Could you check a few things on this model? Use its own coordinates, in mm. Face numbers are marked on the shaded views. Round coordinates to 2 decimals unless told otherwise and drop trailing zeros. Write each loop counter-clockwise with the first axis right and the second up, starting at its lowest first coordinate (ties: lowest second). Pieces come first, ordered by that corner, then holes. Notation, with made-up numbers: (-37, 25.5) -> (-22, 25.5) arc R12 cw to (-22, 40.5) -> close; hole circle Ø2 at (5, 84). An arc over 180 degrees is marked (long way). One line per question, with ' | ' between items. Start each with the question number.
1. Imagine slicing it at A-A, the plane x = 0. List the corners of the cut face in (y, z) for me.
2. Imagine slicing it at B-B, the plane y = 0. List the corners of the cut face in (x, z) for me.
3. For pin 1 Ø2 at (y, z) = (0, 0) entering from +X, with a flat end and sliding along its axis, tell me the tip position at first contact or that it passes through.
4. Thinking about a two-plate mould opening in X: for the marked faces 1, 2 and 3, which applies, released by +X, released by -X, zero draft, split by the parting line, or undercut?
5. If I drill on line 1 along X through (y, z) = (-1.75, 10); line 2 along Z through (x, y) = (0, 1.25); line 3 along Z through (x, y) = (-1.5, -3.5), over which ranges is the centre line in solid material (lowest first)? Write a range as [from, to].
6. Imagine slicing it at C-C, the plane z = 0. List the corners of the cut face in (x, y) for me, and give its area (3 significant figures).
7. Imagine slicing it at D-D, the plane x = -2.5. List the corners of the cut face in (y, z) for me, and give its area (3 significant figures).
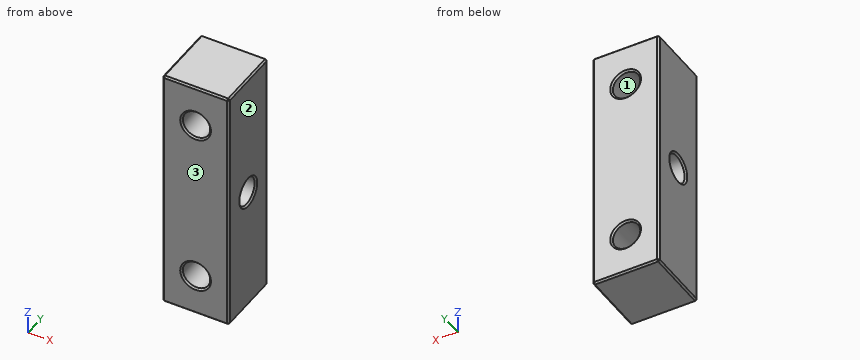
from build123d import *

# Parameters (mm, degrees)
SKETCH_1_W         = 8
SKETCH_1_H         = 8
EXTRUDE_1_DEPTH    = 15
HOLE_WIZARD_M4_1_D = 3.3
HOLE_WIZARD_M4_2_D = 3.3
CHAMFER_1_SIZE     = 0.2


with BuildPart() as part:
    # 草图1 → 凸台-拉伸1 (new, symmetric)
    with BuildSketch(Plane.XY):
        Rectangle(SKETCH_1_W, SKETCH_1_H)
    extrude(amount=EXTRUDE_1_DEPTH, both=True)

    # M4 螺纹孔1 (through all)
    with Locations(Plane(origin=(4, 0, 0), x_dir=(0, 0, -1), z_dir=(1, 0, 0))):
        with Locations((0, 0)):
            Hole(HOLE_WIZARD_M4_1_D / 2)

    # M4 螺纹孔2 (through all)
    with Locations(Plane(origin=(0, 4, 0), x_dir=(1, 0, 0), z_dir=(0, 1, 0))):
        with Locations((0, -10), (0, 10)):
            Hole(HOLE_WIZARD_M4_2_D / 2)

    # 倒角1
    chamfer_1_edges = [part.edges().sort_by_distance(p)[0] for p in [
        (-4, 0, 15),
        (4, 0, -1.65),
        (-4, 0, -1.65),
        (0, -4, 15),
        (1.65, 4, -10),
        (1.65, -4, -10),
        (1.65, 4, 10),
        (1.65, -4, 10),
        (4, 0, 15),
        (0, -4, -15),
        (-4, 0, -15),
        (0, 4, -15),
        (4, 0, -15),
        (4, -4, 0),
        (-4, -4, 0),
        (-4, 4, 0),
        (4, 4, 0),
        (0, 4, 15),
    ]]
    chamfer(chamfer_1_edges, length=CHAMFER_1_SIZE)


solid = part.part
Geometry results:
1) outline: (-4, -14.8) -> (-3.8, -15) -> (3.8, -15) -> (4, -14.8) -> (4, -11.85) -> (3.8, -11.65) -> (-3.8, -11.65) -> (-4, -11.85) -> close; (-4, -8.15) -> (-3.8, -8.35) -> (3.8, -8.35) -> (4, -8.15) -> (4, 8.15) -> (3.8, 8.35) -> (-3.8, 8.35) -> (-4, 8.15) -> close; (-4, 11.85) -> (-3.8, 11.65) -> (3.8, 11.65) -> (4, 11.85) -> (4, 14.8) -> (3.8, 15) -> (-3.8, 15) -> (-4, 14.8) -> close; hole circle Ø3.3 at (0, 0)
2) outline: (-4, -14.8) -> (-3.8, -15) -> (3.8, -15) -> (4, -14.8) -> (4, -1.85) -> (3.8, -1.65) -> (-3.8, -1.65) -> (-4, -1.85) -> close; (-4, 1.85) -> (-3.8, 1.65) -> (3.8, 1.65) -> (4, 1.85) -> (4, 14.8) -> (3.8, 15) -> (-3.8, 15) -> (-4, 14.8) -> close; hole circle Ø3.3 at (0, -10); hole circle Ø3.3 at (0, 10)
3) pin 1: passes through
4) face 1: undercut | face 2: released by +X | face 3: zero draft
5) line 1: x = [-4, -1.65], [1.65, 4] | line 2: z = [-15, -11.65], [-8.35, -1.08], [1.08, 8.35], [11.65, 15] | line 3: z = [-15, -10.69], [-9.31, 9.31], [10.69, 15]
6) outline: (-4, -3.8) -> (-3.8, -4) -> (3.8, -4) -> (4, -3.8) -> (4, -1.85) -> (3.8, -1.65) -> (-3.8, -1.65) -> (-4, -1.85) -> close; (-4, 1.85) -> (-3.8, 1.65) -> (3.8, 1.65) -> (4, 1.85) -> (4, 3.8) -> (3.8, 4) -> (-3.8, 4) -> (-4, 3.8) -> close | area: 37.4 mm2
7) outline: (-4, -14.8) -> (-3.8, -15) -> (3.8, -15) -> (4, -14.8) -> (4, 14.8) -> (3.8, 15) -> (-3.8, 15) -> (-4, 14.8) -> close; hole circle Ø3.3 at (0, 0) | area: 231 mm2
